Verification items for this drawing (mm, ordinates from the low corner). Round coordinates to 2 decimals unless told otherwise and drop trailing zeros. Loops run counter-clockwise (first coordinate to the right, second up) from the corner with the lowest first, then second, coordinate; pieces in that order, holes last. Notation, with made-up numbers: (70.25, 68) -> (82.25, 68) arc R24 ccw to (82.25, 87) -> close; hole circle Ø7 at (18, -36.5). An arc over 180 degrees is marked (long way). One line per question, with ' | ' between items.
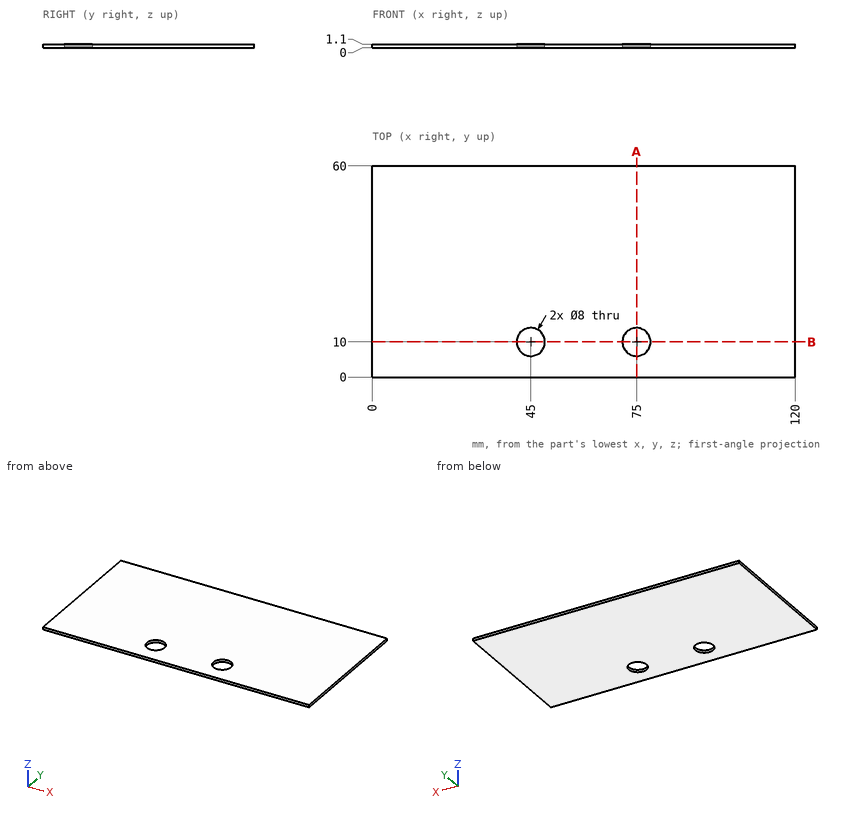
(1) Sectioned sample at A-A, the plane x = 75. Record the cut outline in (y, z), and give its area (3 significant figures).
Answer:
outline: (0, 0) -> (6, 0) -> (6, 1.1) -> (0, 1.1) -> close; (14, 0) -> (60, 0) -> (60, 1.1) -> (14, 1.1) -> close | area: 57.2 mm2
(2) Sectioned sample at B-B, the plane y = 10. Record the cut outline in (x, z).
Answer:
outline: (0, 0) -> (41, 0) -> (41, 1.1) -> (0, 1.1) -> close; (49, 0) -> (71, 0) -> (71, 1.1) -> (49, 1.1) -> close; (79, 0) -> (120, 0) -> (120, 1.1) -> (79, 1.1) -> close
(3) Scan lines: probe 1 along Y at (x, z) = (45, 0.85); probe 2 along Y at (x, z) = (78, 0.65). Record each from-to range of solid material in increasing order.
Answer:
probe 1: y = 0 to 6, 14 to 60 | probe 2: y = 0 to 7.35, 12.65 to 60
(4) Go/stop test with flat-tipped pins: pin 1 (9 mm diameter, centred on x = 45, y = 10, fed in from +Z); pin 2 (7 mm diameter, centred on x = 75, y = 10, fed in from +Z). Record where each tip stops, or that it passes through.
Answer:
pin 1: stops at z = 1.1 | pin 2: passes through
